Verification items for the finished model (mm, model axes). Face numbers are marked on the shaded views. A direction names the side the tool comes from. Coordinates: 2 decimals unless noted, no trailing zeros. Loops run counter-clockwise (first coordinate to the right, second up) from the corner with the lowest first, then second, coordinate; pieces in that order, holes last.
Q1. Sectioned sample at C-C (z = -18.5). Enter the section's corners in (x, y).
Q2. Go/stop test with flat-tipped pins: P1, Ø13, axis at x = 0, z = -60, coming from the +Y side; P2, Ø3, axis at x = 10.5, y = 4, coming from the +Z side. Record where each tip stops, or that it passes through.
Q3. Access from +Z, -Z, +X, -X, +Y, -Y to the whole of each face (thin tool, end or side, straight path). Record for the marked faces 4 and 5.
Q4. Material ranges on probe 1 along Y at (x, z) = (6, -20.5); probe 2 along X at (y, z) = (2.75, 0); probe 3 along Z at (x, y) = (0, 2.1), recorded low to high.
Q5. Sectioned sample at D-D (y = 1.75). Count the separate pieces of the cut face and the enclosed holes in it, then the cut area to 3 significant figures.
Q6. Mould release check, pull along Y, two halves, no side actions. Record for the marked faces 1, 2 and 3: +Y half, -Y half, draft (parallel to the pull), parting line (faces both ways), or undercut.
Q7. Sectioned sample at B-B (z = -60). Enter the section's corners in (x, y), then the cut area to 3 significant figures.
Q8. Sectioned sample at A-A (x = 0). Enter the section's corners in (y, z).
Autodesk Inventor part; units mm, degrees
ref_plane "YZ Plane" through (0, 0, 0) normal (1, 0, 0) x (0, 1, 0)
ref_plane "XZ Plane" through (0, 0, 0) normal (0, 1, 0) x (-1, 0, 0)
ref_plane "XY Plane" through (0, 0, 0) normal (0, 0, 1) x (1, 0, 0)
sketch "Sketch1" plane through (0, 0, 0) normal (0, 1, 0) x (-1, 0, 0)
  circle A0 centre (0, 0) radius 8
  arc A1 (11, 0) -> (-11, 0) centre (0, 0) ccw
  line L0 (-11, 0) -> (-18.0711, -7.0711)
  line L1 (-11, 0) -> (-1, 0) construction
  line L2 (-18.0711, -7.0711) -> (-18.0711, -32.4711)
  line L3 (11, 0) -> (18.0711, -7.0711)
  line L4 (11, 0) -> (21, 0) construction
  line L5 (18.0711, -7.0711) -> (18.0711, -32.4711)
  line L6 (18.0711, -32.4711) -> (-18.0711, -32.4711)
  dimension "d0" = 16
  dimension "d2" = 10
  dimension "d3" = 135
  dimension "d4" = 25.4
  dimension "d5" = 10
  dimension "d6" = 45
extrude "Extrusion1" add sketch "Sketch1" along normal blind 24
sketch "Sketch2" plane through (18.0711, 0, -32.4711) normal (0, 0, -1) x (-1, 0, 0)
  line L0 (7.0711, 0) -> (0, 0)
  line L1 (0, 24) -> (36.1421, 24)
  line L2 (0, 0) -> (36.1421, 0)
  line L3 (36.1421, 0) -> (36.1421, 24)
  line L4 (36.1421, 24) -> (0, 24)
  line L5 (0, 24) -> (0, 0)
  point P0 (18.0711, 0)
extrude "Extrusion2" add sketch "Sketch2" along normal blind 60
sketch "Sketch3" plane through (18.0711, 0, -7.0711) normal (1, 0, 0) x (0, 0, -1)
  line L0 (-7.0711, 0) -> (-7.0711, 24)
  line L1 (52.9289, 12) -> (52.9289, 20)
  line L2 (52.9289, 12) -> (52.9289, 4)
  line L3 (52.9289, 4) -> (-7.0711, 4)
  line L4 (-7.0711, 4) -> (-7.0711, 20)
  line L5 (-7.0711, 20) -> (52.9289, 20)
  line L6 (-18.0711, 0) -> (-18.0711, 24)
  line L7 (-7.0711, 20) -> (-18.0711, 20)
  line L8 (-18.0711, 20) -> (-18.0711, 4)
  line L9 (-18.0711, 4) -> (-7.0711, 4)
  line L10 (-7.0711, 4) -> (-7.0711, 20)
  line L11 (67.9289, 12) -> (67.9289, 20)
  line L12 (67.9289, 20) -> (52.9289, 20)
  line L13 (67.9289, 12) -> (67.9289, 4)
  line L14 (67.9289, 4) -> (52.9289, 4)
  dimension "d13" = 8
extrude "Extrusion3" cut sketch "Sketch3" against normal through all
sketch "Sketch4" plane through (0, 24, 0) normal (0, 1, 0) x (1, 0, 0)
  circle A0 centre (0, 60) radius 8
  point P0 (0, 0)
  dimension "d18" = 16
extrude "Extrusion4" cut sketch "Sketch4" against normal through all
properties part number "Joint1"
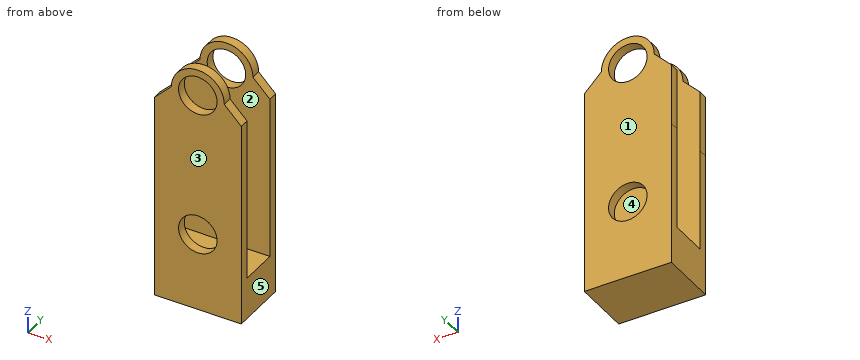
Geometry check:
1. outline: (-18.07, 0) - (18.07, 0) - (18.07, 4) - (-18.07, 4) - close; (-18.07, 20) - (18.07, 20) - (18.07, 24) - (-18.07, 24) - close
2. P1: passes through
2. P2: stops at z = 6.32
3. face 4: +Z, +X, -X
3. face 5: +Z, -Z, +X, +Y, -Y
4. probe 1: y = 0 to 4, 20 to 24
4. probe 2: x = -11 to -8, 8 to 11
4. probe 3: z = -92.47 to -68, -52 to -8, 8 to 11
5. separate pieces: 1
5. enclosed holes: 2
5. area: 3,080 mm2
6. face 1: +Y half
6. face 2: undercut
6. face 3: -Y half
7. outline: (-18.07, 0) - (-8, 0) - (-8, 4) - (-18.07, 4) - close; (-18.07, 20) - (-8, 20) - (-8, 24) - (-18.07, 24) - close; (8, 0) - (18.07, 0) - (18.07, 4) - (8, 4) - close; (8, 20) - (18.07, 20) - (18.07, 24) - (8, 24) - close
7. area: 161 mm2
8. outline: (0, -92.47) - (24, -92.47) - (24, -68) - (20, -68) - (20, -75) - (4, -75) - (4, -68) - (0, -68) - close; (0, -52) - (4, -52) - (4, -8) - (0, -8) - close; (0, 8) - (4, 8) - (4, 11) - (0, 11) - close; (20, -52) - (24, -52) - (24, -8) - (20, -8) - close; (20, 8) - (24, 8) - (24, 11) - (20, 11) - close
